The listing builds one solid part. Answer for the finished solid, in the listing's coordinates (mm). A direction names the side the tool comes from. Give positions to 0.01 mm unless a question says otherwise; leave off trailing zeros. Write each loop counter-clockwise with the first axis right and the second up, starting at its lowest first coordinate (ties: lowest second). Pieces come first, ordered by that corner, then holes. Notation, with made-up numbers: (-21, 85.25) - (31, 85.25) arc R24 cw to (31, 118.25) - close; hole circle Ø3 at (54, 62). An arc over 180 degrees is marked (long way). Write each question's results on one line, items separated by ' | '. Start each with the question number.
Q1. For faces 1 (the face through (0, 0, -37.5)), 2 (the face through (0, -3, 25)), determine the directions among +Z, -Z, +X, -X, +Y, -Y from which every point of the face is accessible in a straight line to the end or side of a thin tool.
Q2. Section D-D (z = 19) is taken. Determine the outline of the cut face in (x, y).
Q3. Flat-ended cylindrical pins translate along their axes: pin 1 Ø3 at (y, z) = (4, -1.5) entering from -X; pin 2 Ø1 at (x, y) = (2, -3.5) entering from +Z. Find the tip coordinate at first contact, or state that the pin passes through.
Q4. Find the intervals of material crossed by probe 1 along Z at (x, y) = (3.25, -1); probe 2 along Y at (x, z) = (4, 3), in increasing order.
Q5. Section C-C (z = -1.5) is taken. Determine the outline of the cut face in (x, y), plus the area to 3 significant figures.
Q6. Section A-A (x = 0) is taken. Determine the outline of the cut face in (y, z).
```python
from build123d import *

# Parameters (mm, degrees)
FILLET1_R     = 0.5
CHAMFER1_SIZE = 0.5


with BuildPart() as part:
    # Sketch1 → Revolve1 (revolve)
    with BuildSketch(Plane(origin=(0, 0, 0), x_dir=(0, 0, -1), z_dir=(1, 0, 0))):
        with BuildLine():
            Line((-37.5, 0), (37.5, 0))
            Line((37.5, 0), (37.5, 5))
            Line((37.5, 5), (-9.5, 5))
            Line((-9.5, 5), (-9.5, 3))
            Line((-9.5, 3), (-12, 3))
            ThreePointArc((-12, 3), (-12.25, 2.75), (-12.5, 3))
            Line((-12.5, 3), (-37.5, 3))
            Line((-37.5, 3), (-37.5, 0))
        make_face()
    revolve(axis=Axis((0, 0, 258.883884114), (0, 0, -1)))

    # Fillet1
    fillet1_edges = [part.edges().sort_by_distance(p)[0] for p in [
        (0, -3, 9.5),
    ]]
    fillet(fillet1_edges, radius=FILLET1_R)

    # Chamfer1
    chamfer1_edges = [part.edges().sort_by_distance(p)[0] for p in [
        (0, -5, -37.5),
        (0, -3, 37.5),
        (0, -5, 9.5),
    ]]
    chamfer(chamfer1_edges, length=CHAMFER1_SIZE)


solid = part.part
```
Answers below:
1) face 1: -Z, +X, -X, +Y, -Y | face 2: +Z
2) outline: circle Ø6 at (0, 0)
3) pin 1: stops at x = -4.33 | pin 2: stops at z = 9.5
4) probe 1: z = -37.5 to 9.51 | probe 2: y = -3 to 3
5) outline: circle Ø10 at (0, 0) | area: 78.5 mm2
6) outline: (-5, -37) - (-4.5, -37.5) - (4.5, -37.5) - (5, -37) - (5, 9) - (4.5, 9.5) - (3.5, 9.5) arc R0.5 cw to (3, 10) - (3, 12) arc R0.25 cw to (3, 12.5) - (3, 37) - (2.5, 37.5) - (-2.5, 37.5) - (-3, 37) - (-3, 12.5) arc R0.25 cw to (-3, 12) - (-3, 10) arc R0.5 cw to (-3.5, 9.5) - (-4.5, 9.5) - (-5, 9) - close
